```python
from build123d import *

# Parameters (mm, degrees)
CROQUIS2_W                   = 20
CROQUIS2_H                   = 16
SALIENTE_EXTRUIR1_DEPTH      = 2
SALIENTE_EXTRUIR2_DEPTH      = 2
CROQUIS4_R                   = 1
SALIENTE_EXTRUIR3_DEPTH      = 3
SALIENTE_EXTRUIR4_DEPTH      = 1
SALIENTE_EXTRUIR4_DEPTH_BACK = 1


with BuildPart() as part:
    # Croquis2 → Saliente-Extruir1 (new body)
    with BuildSketch(Plane.XY):
        Rectangle(CROQUIS2_W, CROQUIS2_H)
    extrude(amount=SALIENTE_EXTRUIR1_DEPTH)

    # Croquis3 → Saliente-Extruir2 (add)
    with BuildSketch(Plane.XY.offset(2)):
        with BuildLine():
            Line((1, -8), (1, -4))
            ThreePointArc((1, -4), (3.764366067, -1.528144202), (7.050666594, 0.190000052))
            ThreePointArc((7.050666594, 0.190000052), (8.85620748, 3.917648534), (5.217391304, 5.896122171))
            ThreePointArc((5.217391304, 5.896122171), (0, 5.203603311), (-5.217391304, 5.896122171))
            ThreePointArc((-5.217391304, 5.896122171), (-8.85620748, 3.917648534), (-7.050666594, 0.190000052))
            ThreePointArc((-7.050666594, 0.190000052), (-3.764366067, -1.528144202), (-1, -4))
            Line((-1, -4), (-1, -8))
            Line((-1, -8), (1, -8))
        make_face()
    extrude(amount=SALIENTE_EXTRUIR2_DEPTH)

    # Croquis4 → Saliente-Extruir3 (add)
    with BuildSketch(Plane.XY.offset(4)):
        with Locations((-6, 3)):
            Circle(CROQUIS4_R)
        with Locations(Location((6, 3, 0), (0, 0, 180))):
            Circle(CROQUIS4_R)
    extrude(amount=SALIENTE_EXTRUIR3_DEPTH)

    # Croquis5 → Saliente-Extruir4 (add, two sides: drawn at the far end of the back side and taken through both)
    with BuildSketch(Plane(origin=(0, 0, 0), x_dir=(0, 0, -1), z_dir=(1, 0, 0)).offset(-SALIENTE_EXTRUIR4_DEPTH_BACK)):
        with BuildLine():
            Line((-4, -8), (-2.00123418, -8))
            ThreePointArc((-2.00123418, -8), (-10.990655722, -16.850952462), (-19.998436931, -8.018685662))
            ThreePointArc((-19.998436931, -8.018685662), (-18.950438256, -6.998395625), (-17.99933798, -8.109566741))
            ThreePointArc((-17.99933798, -8.109566741), (-10.94456846, -15.094975828), (-4, -8))
        make_face()
    extrude(amount=SALIENTE_EXTRUIR4_DEPTH + SALIENTE_EXTRUIR4_DEPTH_BACK)


solid = part.part
```
The model under review builds one solid part; all positions refer to its coordinate system, in mm. A direction names the side the tool comes from. Round coordinates to 2 decimals unless told otherwise and drop trailing zeros. Loops run counter-clockwise (first coordinate to the right, second up) from the corner with the lowest first, then second, coordinate; pieces in that order, holes last.
1) Tool access review of faces 5 (the face through (-10, 0, 1)), 6 (the face through (-6.737, 3.676, 5.479)), 7 (the face through (-1, -15, 8)), 8 (the face through (6, 3, 7)), 9 (the face through (3.72, -1.56, 2.99)): name each direction out of +Z, -Z, +X, -X, +Y, -Y from which nothing blocks a thin tool from reaching the whole face with its end or side.
Values follow:
face 5: +Z, -Z, -X, +Y, -Y
face 6: +Z
face 7: +Z, -X, -Y
face 8: +Z, +X, -X, +Y, -Y
face 9: +Z, +X, -Y
2) Consider section B-B on y = 3. State the section outline as (x, z) points, then the cut area to 3 significant figures.
Values follow:
outline: (-10, 0) - (10, 0) - (10, 2) - (9, 2) - (9, 4) - (7, 4) - (7, 7) - (5, 7) - (5, 4) - (-5, 4) - (-5, 7) - (-7, 7) - (-7, 4) - (-9, 4) - (-9, 2) - (-10, 2) - close
area: 88.0 mm2
3) Consider section A-A on y = -8.75. State the section outline as (x, z) points.
Values follow:
outline: (-1, 2.05) - (1, 2.05) - (1, 4.03) - (-1, 4.03) - close; (-1, 17.97) - (1, 17.97) - (1, 19.95) - (-1, 19.95) - close
4) Consider section C-C on z = 6. State the section outline as (x, y) points, then the cut area to 3 significant figures.
Values follow:
outline: circle Ø2 at (-6, 3); (-1, -15.33) - (1, -15.33) - (1, -12.99) - (-1, -12.99) - close; circle Ø2 at (6, 3)
area: 11.0 mm2
5) Consider section D-D on x = 3.75. State the section outline as (y, z) points, then the cut area to 3 significant figures.
Values follow:
outline: (-8, 0) - (8, 0) - (8, 2) - (5.56, 2) - (5.56, 4) - (-1.54, 4) - (-1.54, 2) - (-8, 2) - close
area: 46.2 mm2
6) The part is to be moulded in two halves that separate along Z. For faces 1 (the face through (8.875, 3.857, 2.986)), 2 (the face through (-0.014, -6.998, 18.973)), 3 (the face through (0, 0, 0)), 4 (the face through (-6, 3, 7)), say which applies: pulls with the +Z half, pulls with the -Z half, needs draft (parallel to the pull), parting line crosses it, or undercut.
Values follow:
face 1: needs draft
face 2: undercut
face 3: pulls with the -Z half
face 4: pulls with the +Z half
7) Wall thickness on line 1 along Z through (x, y) = (-5.25, -5.75); line 2 along Z through (x, y) = (3.25, -0.5); line 3 along X through (y, z) = (-6.5, 3.5): over which ranges is each line inside the solid? List them lowest first.
Values follow:
line 1: z = 0 to 2
line 2: z = 0 to 4
line 3: x = -1 to 1
8) Clearance check with flat-ended pins moving along their axes: P1, Ø7, axis at x = -4.5, y = -4.5, coming from the +Z side; P2, Ø1, axis at x = -6, y = 3.5, coming from the +Z side; P3, Ø0.6, axis at x = 1, z = 1, coming from the -Y side; P4, Ø8, axis at x = -6.5, z = 12, coming from the -Y side. State where each tip first meets the part, or that it passes through.
Values follow:
P1: stops at z = 4
P2: stops at z = 7
P3: stops at y = -8
P4: passes through
